Input: dimensioned drawing with shaded views. Units: mm. Origin: part minimum x, y, z. Round coordinates to 2 decimals unless told otherwise and drop trailing zeros. Write each loop counter-clockwise with the first axis right and the second up, starting at its lowest first coordinate (ties: lowest second). Pieces come first, ordered by that corner, then holes. Notation, with made-up numbers: (17.5, 65.25) - (75.5, 65.25) arc R19 ccw to (75.5, 85.25) - close; hole circle Ø4 at (-28.5, 8.5). An arc over 180 degrees is marked (long way). Use one line per item in the form item = value.
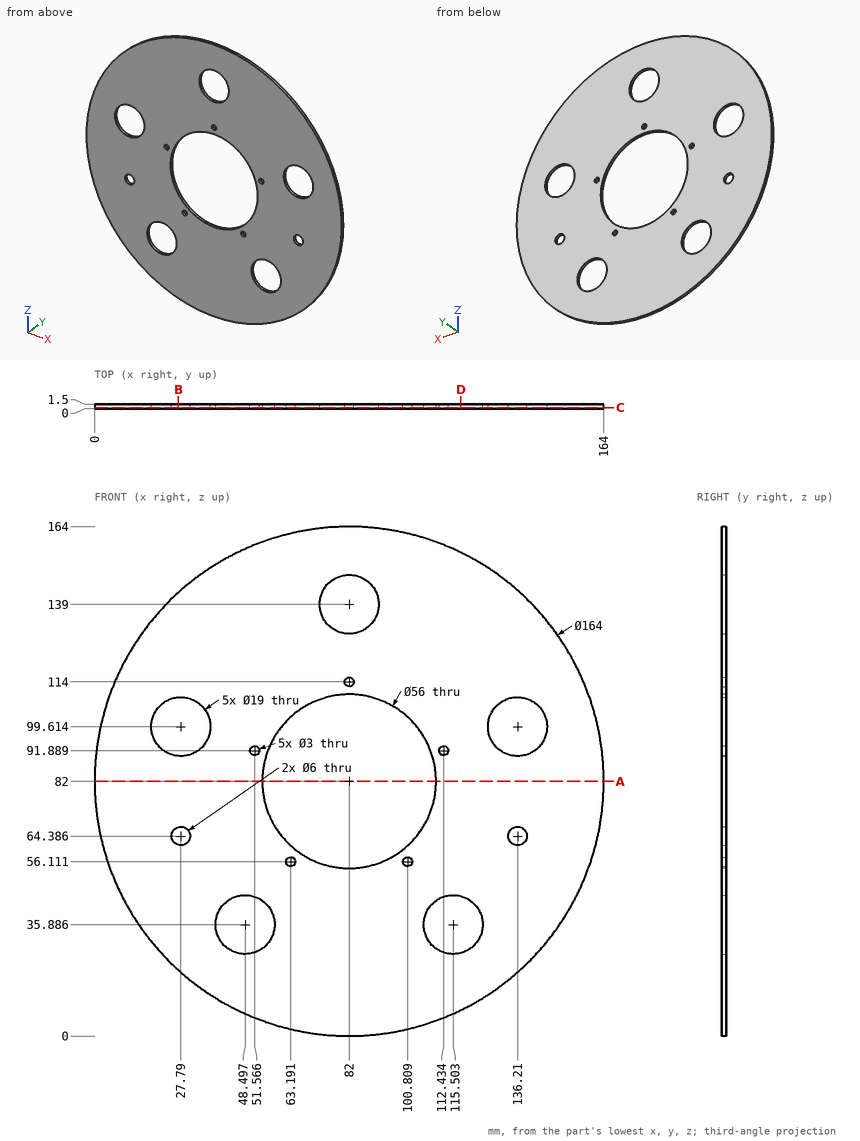
(1) Cut plane D-D on x = 118. Output: boundary loops of the cut face in (y, z) (1 decimal).
Derived:
outline = (0, 8.3) - (1.5, 8.3) - (1.5, 26.7) - (0, 26.7) - close; (0, 45.1) - (1.5, 45.1) - (1.5, 155.7) - (0, 155.7) - close
(2) Cut plane A-A on z = 82. Output: boundary loops of the cut face in (x, y), then the cut area to 3 significant figures.
Derived:
outline = (0, 0) - (54, 0) - (54, 1.5) - (0, 1.5) - close; (110, 0) - (164, 0) - (164, 1.5) - (110, 1.5) - close
area = 162 mm^2
(3) Material intervals for L1, parallel to Z at x = 82, y = 0.5; L2, parallel to X at y = 0.4, z = 32.5 (1 decimal); L3, parallel to X at y = 1.4, z = 95.5 (1 decimal), sorted ascending.
Derived:
L1 = 0 to 54, 110 to 112.5, 115.5 to 129.5, 148.5 to 164
L2 = 16.6 to 39.6, 57.4 to 106.6, 124.4 to 147.4
L3 = 1.1 to 19.2, 36.4 to 57.5, 106.5 to 127.6, 144.8 to 162.9
(4) Cut plane C-C on y = 0.35. Count the separate pieces of the cut face and the enclosed holes in it, then the cut area to 3 significant figures.
Derived:
separate_pieces = 1
enclosed_holes = 13
area = 17,200 mm^2
(5) First-contact query: pin 1 Ø5 at (x, z) = (100.81, 56.11) entering from +Y; pin 2 Ø1.8 at (x, z) = (51.57, 91.89) entering from -Y. Flat tips, straight axial feed; report the tip coordinate or a pass-through.
Derived:
pin_1 = 1.5
pin_2 = through
(6) Cut plane B-B on x = 27. Output: boundary loops of the cut face in (y, z).
Derived:
outline = (0, 21.18) - (1.5, 21.18) - (1.5, 61.49) - (0, 61.49) - close; (0, 67.28) - (1.5, 67.28) - (1.5, 90.15) - (0, 90.15) - close; (0, 109.08) - (1.5, 109.08) - (1.5, 142.82) - (0, 142.82) - close
